```python
from build123d import *

# Parameters (mm, degrees)
BOSS_EXTRUDE1_DEPTH = 152.146
SKETCH2_W           = 2.629781943
SKETCH2_H           = 4.979405242
SKETCH2_W_2         = 2.539494313
SKETCH2_H_2         = 5.192930254
BOSS_EXTRUDE3_DEPTH = 2.032
SKETCH3_W           = 2.60862661
SKETCH3_H           = 5.045368892
SKETCH3_W_2         = 2.568412546
BOSS_EXTRUDE4_DEPTH = 1.651


with BuildPart() as part:
    # Sketch1 → Boss-Extrude1 (new body)
    with BuildSketch(Plane(origin=(0, 0, 0), x_dir=(0, 0, -1), z_dir=(1, 0, 0))):
        with BuildLine():
            Line((-32.603582083, 33.04768703), (-6.580220299, 33.04768703))
            ThreePointArc((-6.580220299, 33.04768703), (-2.866044415, 32.492434763), (0.523359095, 30.875229944))
            Line((0.523359095, 30.875229944), (13.81460794, 7.851288488))
            ThreePointArc((13.81460794, 7.851288488), (14.944302174, 0.295801394), (12.265554132, -6.858631022))
            Line((12.265554132, -6.858631022), (2.114134999, -21.333695036))
            ThreePointArc((2.114134999, -21.333695036), (-2.423671509, -25.308819533), (-8.283736886, -26.741626725))
            Line((-8.283736886, -26.741626725), (-41.665173314, -26.741626725))
            Line((-41.665173314, -26.741626725), (-41.665173314, -25.127558449))
            Line((-41.665173314, -25.127558449), (-7.009997937, -25.127558449))
            ThreePointArc((-7.009997937, -25.127558449), (-2.763170648, -24.353946154), (0.523359095, -21.555242836))
            Line((0.523359095, -21.555242836), (10.572249768, -6.954220772))
            ThreePointArc((10.572249768, -6.954220772), (13.138578862, 0.45392413), (11.185206305, 8.046749136))
            Line((11.185206305, 8.046749136), (-1.796106944, 29.486000218))
            ThreePointArc((-1.796106944, 29.486000218), (-3.505733028, 30.516318699), (-5.469291084, 30.875229944))
            Line((-5.469291084, 30.875229944), (-32.603582083, 30.875229944))
            Line((-32.603582083, 30.875229944), (-32.603582083, 33.04768703))
        make_face()
    extrude(amount=BOSS_EXTRUDE1_DEPTH)

    # Sketch2 → Boss-Extrude3 (add)
    with BuildSketch(Plane(origin=(0, 33.04768703, 0), x_dir=(1, 0, 0), z_dir=(0, 1, 0))):
        with Locations((-1.314890972, -25.618719559)):
            Rectangle(SKETCH2_W, SKETCH2_H)
        with Locations((153.415747157, -25.725482065)):
            Rectangle(SKETCH2_W_2, SKETCH2_H_2)
    extrude(amount=-BOSS_EXTRUDE3_DEPTH)

    # Sketch3 → Boss-Extrude4 (add)
    with BuildSketch(Plane.XZ.offset(26.741626725)):
        with Locations((-1.304313305, 33.959702232)):
            Rectangle(SKETCH3_W, SKETCH3_H)
        with Locations((153.430206273, 33.959702232)):
            Rectangle(SKETCH3_W_2, SKETCH3_H)
    extrude(amount=-BOSS_EXTRUDE4_DEPTH)


solid = part.part
```
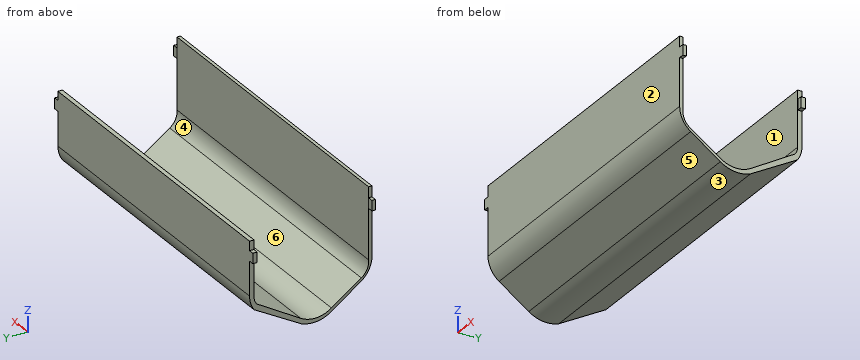
Geometry: final body of the model. Coordinates: model frame, mm. Face numbers are marked on the shaded views. A direction names the side the tool comes from. Coordinates: 2 decimals unless noted, no trailing zeros. Order: outer loops, then holes, each group sorted by start corner. A loop starts at its lowest first (then second) coordinate and runs counter-clockwise, first axis right, second up. Notation, with made-up numbers: M 60,-34 L 119,-34 A9 cw 119,-27 Z; hole C -11.5,-4.75 d4. An arc over 180 degrees is marked long. Answer as CSV lines item,"result".
Q1. Set-up query: the marked faces 1 and 2. Return all of +Z, -Z, +X, -X, +Y, -Y with unobstructed straight access to the full face (end or side cutting, diameter ignored); none if empty.
Answers:
face 1,"+Z, +X, -X"
face 2,"+Z, -Z, +X, -X, -Y"
Q2. Section B-B on x = 126. Return the cut outline in (y, z).
Answers:
outline,"M -26.74,8.28 A12.7 ccw -21.33,-2.11 L -6.86,-12.27 A15.24 ccw 7.85,-13.81 L 30.88,-0.52 A12.7 ccw 33.05,6.58 L 33.05,32.6 L 30.88,32.6 L 30.88,5.47 A5.55 cw 29.49,1.8 L 8.05,-11.19 A13.59 cw -6.95,-10.57 L -21.56,-0.52 A8.31 cw -25.13,7.01 L -25.13,41.67 L -26.74,41.67 Z"
Q3. First-contact query: P1, Ø10, axis at y = -20, z = 35.5, coming from the +X side; P2, Ø1.8, axis at y = -25.5, z = 40, coming from the +X side; P3, Ø1.5, axis at x = 124, y = 26.5, coming from the -Z side; P4, Ø1, axis at x = 131, y = 25.5, coming from the +Z side. Flat tips, straight axial feed; report the tip coordinate or a pass-through.
Answers:
P1,"passes through"
P2,"stops at x = 152.15"
P3,"stops at z = -3.48"
P4,"stops at z = -0.31"
Q4. Section A-A on z = 21.5. Return the cut outline in (x, y), and give its area (3 significant figures).
Answers:
outline,"M 0,-26.74 L 152.15,-26.74 L 152.15,-25.13 L 0,-25.13 Z; M 0,30.88 L 152.15,30.88 L 152.15,33.05 L 0,33.05 Z"
area,"576 mm^2"
Q5. Section D-D on z = -8. Return the cut outline in (x, y), and give its area (3 significant figures).
Answers:
outline,"M 0,-12.94 L 152.15,-12.94 L 152.15,-10.69 L 0,-10.69 Z; M 0,13.31 L 152.15,13.31 L 152.15,17.92 L 0,17.92 Z"
area,"1,040 mm^2"
Q6. Draft query along Y for the marked faces 3, 4, 5 and 6. Return one class per face: pulls with the +Y half, pulls with the -Y half, needs draft (parallel to the pull), parting line crosses it, or undercut.
Answers:
face 3,"parting line crosses it"
face 4,"undercut"
face 5,"pulls with the -Y half"
face 6,"undercut"
Q7. Section C-C on y = -9. Return the cut outline in (x, z), and give its area (3 significant figures).
Answers:
outline,"M 0,-10.76 L 152.15,-10.76 L 152.15,-9.16 L 0,-9.16 Z"
area,"243 mm^2"
Q8. Line query: probe 1 along Y at (x, z) = (133, 20); probe 2 along Y at (x, z) = (42, -10); probe 3 along Y at (x, z) = (5, 36.5). Output: solid intervals per line, ascending. Write a range as [from, to].
Answers:
probe 1,"y = [-26.74, -25.13], [30.88, 33.05]"
probe 2,"y = [-10.09, -7.79], [10, 14.46]"
probe 3,"y = [-26.74, -25.13]"
